Here's how the part is built. I have some questions about the finished solid (model axes, mm). A direction names the side the tool comes from. Give positions to 0.01 mm unless a question says otherwise; leave off trailing zeros. Order: outer loops, then holes, each group sorted by start corner. A loop starts at its lowest first (then second) coordinate and runs counter-clockwise, first axis right, second up.
from build123d import *

# Parameters (mm, degrees)
IZIM12_R                = 1.6
KES_EKSTR_ZYON1_DEPTH   = 133.664991614
DAIRESEL_KAPLAMA1_COUNT = 6
KES_EKSTR_ZYON2_START   = 32
IZIM13_R                = 1.49
KES_EKSTR_ZYON2_DEPTH   = 5
DAIRESEL_KAPLAMA2_COUNT = 4
IZIM14_R                = 1.6
KES_EKSTR_ZYON3_DEPTH   = 133.664991614
DAIRESEL_KAPLAMA3_COUNT = 4
IZIM15_R                = 3
KES_EKSTR_ZYON5_DEPTH   = 36
DAIRESEL_KAPLAMA4_COUNT = 4
RADYUS1_R               = 15


with BuildPart() as part:
    # Çizim1 → Döndür1 (revolve)
    with BuildSketch(Plane.XY, mode=Mode.PRIVATE) as d_nd_r1_sk:
        Polygon((-60, 40), (-60, 37), (-70, 37), (-70, 22), (-120, 22), (-120, 4), (-118, 4), (-118, 18.2), (-66, 18.2), (-66, 29.2), (-60, 29.2), (-52, 36), (-30, 36), (-30, 38), (-20, 38), (-20, 40), align=None)
    revolve(d_nd_r1_sk.sketch.rotate(Axis((-88.99, 0, 0), (1, 0, 0)), 90), axis=Axis((-88.99, 0, 0), (1, 0, 0)))

    # Çizim12 → Kes-Ekstrüzyon1 (cut, through all)
    with BuildSketch(Plane(origin=(0, 0, 0), x_dir=(0, 0, -1), z_dir=(1, 0, 0))):
        with Locations((12.5, 0)):
            Circle(IZIM12_R)
    kes_ekstr_zyon1 = extrude(amount=-KES_EKSTR_ZYON1_DEPTH, mode=Mode.SUBTRACT)

    # Dairesel Kaplama1: Kes-Ekstrüzyon1 ×6 about axis
    dairesel_kaplama1_axis = Axis((0, 0, 0), (1, 0, 0))
    for i in range(1, DAIRESEL_KAPLAMA1_COUNT):
        add(kes_ekstr_zyon1.rotate(dairesel_kaplama1_axis, i * 360 / DAIRESEL_KAPLAMA1_COUNT), mode=Mode.SUBTRACT)

    # Çizim13 → Kes-Ekstrüzyon2 (cut)
    with BuildSketch(Plane.XY.offset(KES_EKSTR_ZYON2_START)):
        with Locations((-65, 0)):
            Circle(IZIM13_R)
    kes_ekstr_zyon2 = extrude(amount=KES_EKSTR_ZYON2_DEPTH, mode=Mode.SUBTRACT)

    # Dairesel Kaplama2: Kes-Ekstrüzyon2 ×4 about axis
    dairesel_kaplama2_axis = Axis((0, 0, 0), (1, 0, 0))
    for i in range(1, DAIRESEL_KAPLAMA2_COUNT):
        add(kes_ekstr_zyon2.rotate(dairesel_kaplama2_axis, i * 360 / DAIRESEL_KAPLAMA2_COUNT), mode=Mode.SUBTRACT)

    # Çizim14 → Kes-Ekstrüzyon3 (cut, through all)
    with BuildSketch(Plane.XY):
        with Locations((-25, 0)):
            Circle(IZIM14_R)
    kes_ekstr_zyon3 = extrude(amount=-KES_EKSTR_ZYON3_DEPTH, mode=Mode.SUBTRACT)

    # Dairesel Kaplama3: Kes-Ekstrüzyon3 ×4 about axis
    dairesel_kaplama3_axis = Axis((-88.99, 0, 0), (1, 0, 0))
    for i in range(1, DAIRESEL_KAPLAMA3_COUNT):
        add(kes_ekstr_zyon3.rotate(dairesel_kaplama3_axis, i * 360 / DAIRESEL_KAPLAMA3_COUNT), mode=Mode.SUBTRACT)

    # Çizim15 → Kes-Ekstrüzyon5 (cut)
    with BuildSketch(Plane(origin=(0, 0, 0), x_dir=(0, 0, -1), z_dir=(1, 0, 0))):
        with Locations((25.809397513, 25.809397513)):
            Circle(IZIM15_R)
    kes_ekstr_zyon5 = extrude(amount=-KES_EKSTR_ZYON5_DEPTH, mode=Mode.SUBTRACT)

    # Dairesel Kaplama4: Kes-Ekstrüzyon5 ×4 about axis
    dairesel_kaplama4_axis = Axis((0, 0, 0), (1, 0, 0))
    for i in range(1, DAIRESEL_KAPLAMA4_COUNT):
        add(kes_ekstr_zyon5.rotate(dairesel_kaplama4_axis, i * 360 / DAIRESEL_KAPLAMA4_COUNT), mode=Mode.SUBTRACT)

    # Radyus1
    radyus1_edges = [part.edges().sort_by_distance(p)[0] for p in [
        (-70, 0, -22),
    ]]
    fillet(radyus1_edges, radius=RADYUS1_R - 0.0001)  # a hair under: the kernel refuses the full size


solid = part.part
Q1. Thinking about a two-plate mould opening in Z: for faces 4 (the face through (-29.67, -27.98, -27.88)), 5 (the face through (-26.27, 0.97, 38.97)), which applies, released by +Z, released by -Z, zero draft, split by the parting line, or undercut?
Filled sheet:
face 4: undercut
face 5: zero draft
Q2. For faces 1 (the face through (-63.624, 34.465, 0.571)), 2 (the face through (-63.624, -34.465, -0.571)), 3 (the face through (-30, 36.2, 0.1)), which set-ups out of +Z, -Z, +X, -X, +Y, -Y let a thin tool reach every point of the face, with its end or its side?
Filled sheet:
face 1: +Y
face 2: -Y
face 3: +X
Q3. I need wall thicknesses on L1, parallel to Y at x = -65.5, z = -1; L2, parallel to Y at x = -119.4, z = 6.25; L3, parallel to Z at x = -67.5, y = -15.5. Which ranges of each line are inside material? Lowest first, please.
Filled sheet:
L1: y = -32 to -29.18, 29.18 to 32
L2: y = -21.09 to -12.43, -9.23 to 9.23, 12.43 to 21.09
L3: z = -33.6 to -9.54, 9.54 to 33.6
Q4. If we section it at C-C on x = -57: List the corners of the cut face in (y, z) for me.
Filled sheet:
outline: circle Ø80 at (0, 0); hole circle Ø63.5 at (0, 0)
Q5. If we section it at B-B on y = 0: Give the number of separate pieces and of enclosed holes in the cut face, plus the area to 3 significant figures.
Filled sheet:
separate pieces: 6
enclosed holes: 0
area: 1,060 mm2
Q6. I'm going to push flat-ended pins straight in: P1, Ø5, axis at x = -25, y = 0, coming from the -Z side; P2, Ø2.5, axis at y = 10.83, z = 6.25, coming from the -X side; P3, Ø3.5, axis at x = -64.5, y = -0.5, coming from the +Z side; P4, Ø2, axis at y = -11, z = -31.5, coming from the +X side. Where does each tip first touch, or does it pass through?
Filled sheet:
P1: stops at z = -40
P2: passes through
P3: stops at z = 37
P4: stops at x = -53.92
Q7. If we section it at A-A on x = -25: List the corners of the cut face in (y, z) for me.
Filled sheet:
outline: (-39.97, -1.6) arc R40 ccw to (-1.6, -39.97) - (-1.6, -37.97) arc R38 cw to (-24.93, -28.68) arc R3 cw to (-28.68, -24.93) arc R38 cw to (-37.97, -1.6) - close; (-39.97, 1.6) - (-37.97, 1.6) arc R38 cw to (-28.68, 24.93) arc R3 cw to (-24.93, 28.68) arc R38 cw to (-1.6, 37.97) - (-1.6, 39.97) arc R40 ccw to start; (1.6, -39.97) arc R40 ccw to (39.97, -1.6) - (37.97, -1.6) arc R38 cw to (28.68, -24.93) arc R3 cw to (24.93, -28.68) arc R38 cw to (1.6, -37.97) - close; (1.6, 37.97) arc R38 cw to (24.93, 28.68) arc R3 cw to (28.68, 24.93) arc R38 cw to (37.97, 1.6) - (39.97, 1.6) arc R40 ccw to (1.6, 39.97) - close
